```python
from build123d import *

# Parameters (mm, degrees)
BOSS_EXTRUDE1_DEPTH = 8
SKETCH4_W           = 10.258234737
SKETCH4_H           = 27
SKETCH4_W_2         = 16
SKETCH4_W_3         = 15
SKETCH4_W_4         = 4
CUT_EXTRUDE1_DEPTH  = 3


with BuildPart() as part:
    # Sketch1 → Boss-Extrude1 (new body)
    with BuildSketch(Plane(origin=(0, 0, 0), x_dir=(1, 0, 0), z_dir=(0, 1, 0))):
        Polygon((-113, -12.62891462), (113, -12.62891462), (128.588457268, 14.37108538), (-128.588457268, 14.37108538), align=None)
    extrude(amount=BOSS_EXTRUDE1_DEPTH)

    # Sketch4 → Cut-Extrude1 (cut)
    with BuildSketch(Plane(origin=(0, 8, 0), x_dir=(1, 0, 0), z_dir=(0, 1, 0))):
        with Locations((-56.935441316, 0.87108538)):
            Rectangle(SKETCH4_W, SKETCH4_H)
        with Locations((-89.935441316, 0.87108538)):
            Rectangle(SKETCH4_W, SKETCH4_H)
        with Locations((-26.935441316, 0.87108538)):
            Rectangle(SKETCH4_W_2, SKETCH4_H)
        with Locations((3.064558684, 0.87108538)):
            Rectangle(SKETCH4_W_2, SKETCH4_H)
        with Locations((33.064558684, 0.87108538)):
            Rectangle(SKETCH4_W_2, SKETCH4_H)
        with Locations((63.064558684, 0.87108538)):
            Rectangle(SKETCH4_W_3, SKETCH4_H)
        with Locations((93.064558684, 0.87108538)):
            Rectangle(SKETCH4_W_4, SKETCH4_H)
    extrude(amount=-CUT_EXTRUDE1_DEPTH, mode=Mode.SUBTRACT)


solid = part.part
```
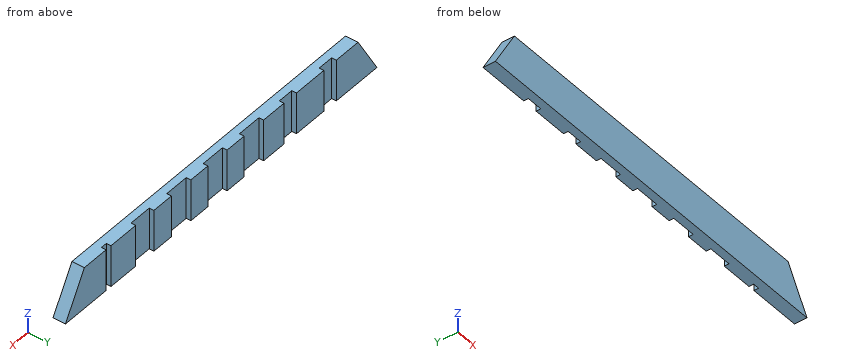
Could you check a few things on this model? Use its own coordinates, in mm. Coordinates: 2 decimals unless noted, no trailing zeros. Write each loop counter-clockwise with the first axis right and the second up, starting at its lowest first coordinate (ties: lowest second). Pieces come first, ordered by that corner, then holes. Notation, with made-up numbers: (7, 44) -> (25, 44) arc R18 cw to (25, 59) -> close; hole circle Ø11 at (-25, 47.25). An arc over 180 degrees is marked (long way). Return JSON: item names as keys, results as strings.
(1) I'm going to push flat-ended pins straight in: pin 1 (0.9 mm diameter, centred on y = 7, z = -2.5, fed in from +X); pin 2 (8 mm diameter, centred on x = -26.5, z = -1, fed in from +Y); pin 3 (4 mm diameter, centred on y = 1.5, z = 7.5, fed in from +X); pin 4 (1 mm diameter, centred on x = -21.5, z = -0.5, fed in from -Y). Where does each tip first touch, or does it pass through?
Numbers:
{"pin 1": "stops at x = 121.99", "pin 2": "stops at y = 5", "pin 3": "stops at x = 117.12", "pin 4": "stops at y = 0"}
(2) I need wall thicknesses on L1, parallel to Y at x = 31.5, z = -12; L2, parallel to X at y = 2.75, z = 0; L3, parallel to X at y = 3.25, z = -13.5. Which ranges of each line are inside material? Lowest first, please.
Numbers:
{"L1": "y = 0 to 5", "L2": "x = -120.29 to 120.29", "L3": "x = -128.09 to 128.09"}
(3) Imagine slicing it at A-A, the plane y = 6.75. Count the separate pieces of the cut face and the enclosed holes in it, then the cut area to 3 significant figures.
Numbers:
{"separate pieces": "8", "enclosed holes": "0", "area": "4,160 mm2"}
(4) Imagine slicing it at C-C, the plane x = 29.5. Please give me the cut outline in (y, z).
Numbers:
{"outline": "(0, -14.37) -> (5, -14.37) -> (5, 12.63) -> (0, 12.63) -> close"}
